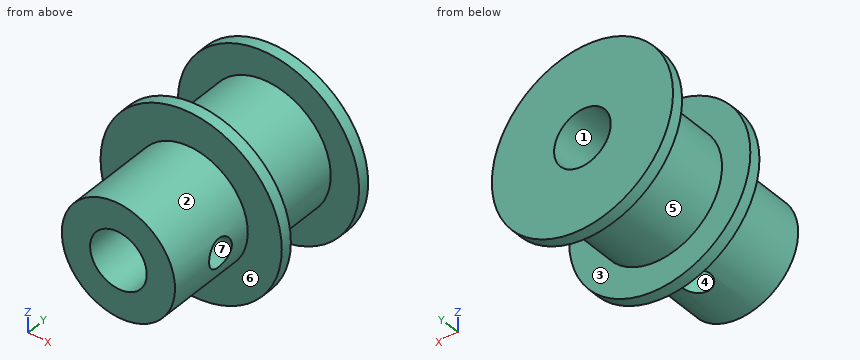
```python
from build123d import *

# Parameters (mm, degrees)
CORTAR_EXTRUIR1_REACH      = 22.839
CORTAR_EXTRUIR1_END_RADIUS = 5
CROQUIS2_R                 = 1.25
MATRIZC1_COUNT             = 2
MATRIZC1_ANGLE             = 90


with BuildPart() as part:
    # Croquis1 → Revolución1 (revolve)
    with BuildSketch(Plane.XY, mode=Mode.PRIVATE) as revoluci_n1_sk:
        Polygon((8, 8), (5, 8), (5, 0), (2.5, 0), (2.5, 17.5), (8, 17.5), (8, 16.5), (5.5, 16.5), (5.5, 9), (8, 9), align=None)
    revolve(revoluci_n1_sk.sketch.rotate(Axis((0, 0, 0), (0, 1, 0)), 90), axis=Axis((0, 0, 0), (0, 1, 0)))

    # Cortar-Extruir1: up to this cylinder (the profile starts inside it)
    cortar_extruir1_end = Plane(origin=(0, 5, 0), z_dir=(0, -1, 0)) * Cylinder(CORTAR_EXTRUIR1_END_RADIUS, 56.678, mode=Mode.PRIVATE)
    # Croquis2 → Cortar-Extruir1 (cut, up to the surface)
    with BuildSketch(Plane.XY, mode=Mode.PRIVATE) as cortar_extruir1_sk1:
        with Locations((0, 5)):
            Circle(CROQUIS2_R)
    cortar_extruir1_tool1 = extrude(cortar_extruir1_sk1.sketch, amount=-CORTAR_EXTRUIR1_REACH, mode=Mode.PRIVATE) & cortar_extruir1_end
    cortar_extruir1 = cortar_extruir1_tool1.solids().sort_by_distance((0, 5, 0))[0]
    add(cortar_extruir1, mode=Mode.SUBTRACT)

    # MatrizC1: Cortar-Extruir1 ×2 about axis
    matrizc1_axis = Axis((0, 0, 0), (0, -1, 0))
    for i in range(1, MATRIZC1_COUNT):
        add(cortar_extruir1.rotate(matrizc1_axis, i * MATRIZC1_ANGLE / (MATRIZC1_COUNT - 1)), mode=Mode.SUBTRACT)


solid = part.part
```
Here's how the part is built. I have some questions about the finished solid (model axes, mm). Face numbers are marked on the shaded views. A direction names the side the tool comes from. Round coordinates to 2 decimals unless told otherwise and drop trailing zeros. Write each loop counter-clockwise with the first axis right and the second up, starting at its lowest first coordinate (ties: lowest second). Pieces come first, ordered by that corner, then holes.
Q1. Will these pins go through, and if not, where does the flat tip stop? P1, Ø1, axis at y = 8, z = -1, coming from the -X side; P2, Ø8, axis at x = 4.5, y = 15.5, coming from the -Z side; P3, Ø1.5, axis at y = 5, z = 0, coming from the -X side.
Q2. Please list where these lines run through material, in increasing order: probe 1 along Y at (x, z) = (4, -5.5); probe 2 along Y at (x, z) = (2.7, 0); probe 3 along Z at (x, y) = (3, 5).
Q3. If we section it at D-D on x = -1: Write out the boundary of the cut face in (y, z).
Q4. If we section it at B-B on x = -6: Write out the boundary of the cut face in (y, z).
Q5. Which directions (+Z, -Z, +X, -X, +Y, -Y) give clear straight access to the entire face, cutting with the end or side of a thin tool? Please do the marked faces 4, 5, 6 and 7.
Q6. If we mould it in two halves opening along X, with no side actions, what happens to the marked faces 1, 2 and 3? For each: +X half, -X half, draft (parallel to the pull), parting line (faces both ways), or undercut.
Q7. If we section it at C-C on y = 5: Write out the boundary of the cut face in (x, z).
Q8. If we section it at A-A on z = 0: Write out the boundary of the cut face in (x, y).
Answer below:
1. P1: stops at x = -7.98
1. P2: stops at z = -7.98
1. P3: stops at x = -5
2. probe 1: y = 8 to 9, 16.5 to 17.5
2. probe 2: y = 0 to 3.75, 6.25 to 17.5
2. probe 3: z = -4 to -1.25, 1.25 to 4
3. outline: (0, -4.9) - (4.25, -4.9) - (4.25, -2.29) - (0, -2.29) - close; (0, 2.29) - (17.5, 2.29) - (17.5, 7.94) - (16.5, 7.94) - (16.5, 5.41) - (9, 5.41) - (9, 7.94) - (8, 7.94) - (8, 4.9) - (0, 4.9) - close; (5.75, -4.9) - (8, -4.9) - (8, -7.94) - (9, -7.94) - (9, -5.41) - (16.5, -5.41) - (16.5, -7.94) - (17.5, -7.94) - (17.5, -2.29) - (5.75, -2.29) - close
4. outline: (8, -5.29) - (9, -5.29) - (9, 5.29) - (8, 5.29) - close; (16.5, -5.29) - (17.5, -5.29) - (17.5, 5.29) - (16.5, 5.29) - close
5. face 4: -Z
5. face 5: none
5. face 6: -Y
5. face 7: +X
6. face 1: undercut
6. face 2: parting line
6. face 3: draft
7. outline: (-1.25, -4.84) - (-1.25, -2.17) arc R2.5 cw (long way) to (2.17, 1.25) - (4.84, 1.25) arc R5 ccw (long way) to start; (1.25, -4.84) arc R5 ccw to (4.84, -1.25) - (2.17, -1.25) arc R2.5 cw to (1.25, -2.17) - close
8. outline: (-8, 8) - (-5, 8) - (-5, 0) - (-2.5, 0) - (-2.5, 17.5) - (-8, 17.5) - (-8, 16.5) - (-5.5, 16.5) - (-5.5, 9) - (-8, 9) - close; (2.5, 0) - (5, 0) - (5, 3.75) - (2.5, 3.75) - close; (2.5, 6.25) - (5, 6.25) - (5, 8) - (8, 8) - (8, 9) - (5.5, 9) - (5.5, 16.5) - (8, 16.5) - (8, 17.5) - (2.5, 17.5) - close
